CAD build for the part. Positions are in the model's coordinates, mm. Face numbers are marked on the shaded views. A direction names the side the tool comes from. Give positions to 0.01 mm unless a question says otherwise; leave off trailing zeros. Order: outer loops, then holes, each group sorted by start corner. A loop starts at its lowest first (then second) coordinate and runs counter-clockwise, first axis right, second up. Notation, with made-up numbers: (15.5, 69) -> (44.5, 69) arc R20 cw to (44.5, 96) -> close; hole circle Ø4 at (10.25, 74). An arc over 180 degrees is marked (long way). Answer as CSV lines item,"result".
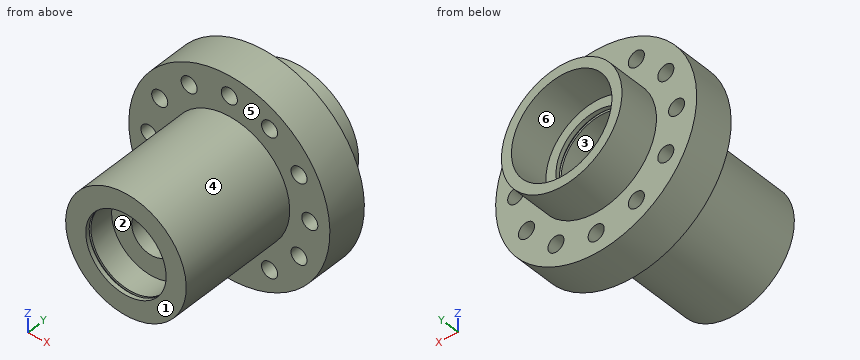
```python
from build123d import *

# Parameters (mm, degrees)
SKETCH2_R           = 4
CUT_EXTRUDE1_DEPTH  = 20
EXTRUDE_THIN1_START = 20
SKETCH3_R           = 30
SKETCH3_R_2         = 25
EXTRUDE_THIN1_DEPTH = 20


with BuildPart() as part:
    # Sketch1 → Revolve1 (revolve)
    with BuildSketch(Plane.XY, mode=Mode.PRIVATE) as revolve1_sk:
        Polygon((50, 80), (20, 80), (20, 78), (21, 78), (21, 77), (20, 77), (20, 65), (10, 65), (10, 15), (20, 15), (20, 3), (21, 3), (21, 2), (20, 2), (20, 0), (30, 0), (30, 60), (50, 60), align=None)
    revolve(revolve1_sk.sketch.rotate(Axis((0, 80, 0), (0, -1, 0)), 90), axis=Axis((0, 80, 0), (0, -1, 0)))

    # Sketch2 → Cut-Extrude1 (cut)
    with BuildSketch(Plane.XZ.offset(-60)):
        with Locations(Location((0, 40, 0), (0, 0, 270))):
            Circle(SKETCH2_R)
        with Locations(Location((20, 34.641016151, 0), (0, 0, 270))):
            Circle(SKETCH2_R)
        with Locations(Location((34.641016151, 20, 0), (0, 0, 270))):
            Circle(SKETCH2_R)
        with Locations(Location((40, 0, 0), (0, 0, 270))):
            Circle(SKETCH2_R)
        with Locations(Location((34.641016151, -20, 0), (0, 0, 270))):
            Circle(SKETCH2_R)
        with Locations(Location((20, -34.641016151, 0), (0, 0, 270))):
            Circle(SKETCH2_R)
        with Locations(Location((0, -40, 0), (0, 0, 270))):
            Circle(SKETCH2_R)
        with Locations(Location((-20, -34.641016151, 0), (0, 0, 270))):
            Circle(SKETCH2_R)
        with Locations(Location((-34.641016151, -20, 0), (0, 0, 270))):
            Circle(SKETCH2_R)
        with Locations(Location((-40, 0, 0), (0, 0, 270))):
            Circle(SKETCH2_R)
        with Locations(Location((-34.641016151, 20, 0), (0, 0, 270))):
            Circle(SKETCH2_R)
        with Locations(Location((-20, 34.641016151, 0), (0, 0, 270))):
            Circle(SKETCH2_R)
    extrude(amount=-CUT_EXTRUDE1_DEPTH, mode=Mode.SUBTRACT)

    # Sketch3 → Extrude-Thin1 (add)
    with BuildSketch(Plane(origin=(0, 80, 0), x_dir=(1, 0, 0), z_dir=(0, 1, 0)).offset(EXTRUDE_THIN1_START)):
        Circle(SKETCH3_R)
        Circle(SKETCH3_R_2, mode=Mode.SUBTRACT)
    extrude(amount=-EXTRUDE_THIN1_DEPTH)


solid = part.part
```
1) Wall check: line 1 along X through (y, z) = (70.75, 0); line 2 along X through (y, z) = (50, 0); line 3 along Z through (x, y) = (-31.5, 62.5). Give the ranges that are in metal, low to high. Write a range as [from, to].
Data:
line 1,"x = [-50, -44], [-36, -20], [20, 36], [44, 50]"
line 2,"x = [-30, -10], [10, 30]"
line 3,"z = [-38.83, -22.48], [-17.52, 17.52], [22.48, 38.83]"
2) Pull direction Z, two halves, no side cores. Call the marked faces 4, 5 and 6: pulls with the +Z half, pulls with the -Z half, needs draft (parallel to the pull), parting line crosses it, or undercut.
Data:
face 4,"parting line crosses it"
face 5,"needs draft"
face 6,"undercut"
3) Pin check, flat tips, straight feed: P1, Ø3, axis at x = 21.5, y = 74, coming from the -Z side; P2, Ø2, axis at y = 13.5, z = 0, coming from the -X side; P3, Ø10.5, axis at x = -20, z = 34.64, coming from the +Y side; P4, Ø6.5, axis at x = -20, z = -34.64, coming from the -Y side. Stop position of each tip, or through.
Data:
P1,"stops at z = -45.83"
P2,"stops at x = -30"
P3,"stops at y = 80"
P4,"passes through"
4) Band-saw the part on C-C, the plane y = 13.5. Write the cut outline in (x, z).
Data:
outline,"circle Ø60 at (0, 0); hole circle Ø40 at (0, 0)"
5) Band-saw the part on A-A, the plane y = 89. Write the cut outline in (x, z).
Data:
outline,"circle Ø60 at (0, 0); hole circle Ø50 at (0, 0)"
6) Which spindle directions (+Z, -Z, +X, -X, +Y, -Y) get a long thin tool onto all of the face, cutting with end or side? Do the marked faces 1, 2 and 3. Say none if no direction does.
Data:
face 1,"+Z, -Z, +X, -X, -Y"
face 2,"-Y"
face 3,"+Y"
7) Band-saw the part on B-B, the plane z = 28.5. Write the cut outline in (x, y).
Data:
outline,"(-41.08, 60) -> (-9.37, 60) -> (-9.37, 0) -> (9.37, 0) -> (9.37, 60) -> (41.08, 60) -> (41.08, 80) -> (9.37, 80) -> (9.37, 100) -> (-9.37, 100) -> (-9.37, 80) -> (-41.08, 80) -> close"
